from build123d import *

# Parameters (mm, degrees)
SKETCH1_R           = 14.2875
BOSS_EXTRUDE1_DEPTH = 11.1125
SKETCH2_R           = 15.875
BOSS_EXTRUDE2_DEPTH = 3.175
SKETCH3_R           = 6.35
CUT_EXTRUDE1_DEPTH  = 26.050327468


with BuildPart() as part:
    # Sketch1 → Boss-Extrude1 (new body)
    with BuildSketch(Plane(origin=(0, 0, 0), x_dir=(1, 0, 0), z_dir=(0, 1, 0))):
        with Locations(Location((0, 0, 0), (0, 0, 270))):
            Circle(SKETCH1_R)
    extrude(amount=BOSS_EXTRUDE1_DEPTH)

    # Sketch2 → Boss-Extrude2 (add)
    with BuildSketch(Plane(origin=(0, 11.1125, 0), x_dir=(1, 0, 0), z_dir=(0, 1, 0))):
        with Locations(Location((0, 0, 0), (0, 0, 270))):
            Circle(SKETCH2_R)
    extrude(amount=-BOSS_EXTRUDE2_DEPTH)

    # Sketch3 → Cut-Extrude1 (cut, through all)
    with BuildSketch(Plane(origin=(0, 11.1125, 0), x_dir=(1, 0, 0), z_dir=(0, 1, 0))):
        with Locations(Location((0, 0, 0), (0, 0, 270))):
            Circle(SKETCH3_R)
    extrude(amount=-CUT_EXTRUDE1_DEPTH, mode=Mode.SUBTRACT)


solid = part.part
Work out the finished part from the listing and answer in its coordinate system (mm). A direction names the side the tool comes from. Coordinates: 2 decimals unless noted, no trailing zeros. Write each loop counter-clockwise with the first axis right and the second up, starting at its lowest first coordinate (ties: lowest second). Pieces come first, ordered by that corner, then holes. Notation, with made-up numbers: M 22.25,40 L 67.25,40 A24 ccw 67.25,76 Z; hole C -40,24 d6. An arc over 180 degrees is marked long. Use one line per item in the form item = value. Start each with the question number.
1. Straight lines are drawn through the part: probe 1 along X at (y, z) = (7.25, 0); probe 2 along X at (y, z) = (8, 0) (3 decimals); probe 3 along Z at (x, y) = (3.5, 8.25). For each, find the intervals that lie inside material, in ascending order. Write a range as from..to.
2. The part is cut by section D-D (x = -7.5). Give the vertices of the cut face in (y, z).
3. The mould has two halves that part along Z. Classify faces 3 (the face through (-3.86, 5.63, -5.04)), 4 (the face through (-15.497, 9.547, -3.441)), 5 (the face through (-7, 11.112, 0)): released by +Z, released by -Z, zero draft, split by the parting line, or undercut.
4. Each of these flat-tipped pins is pushed along its axis until it touches: P1, Ø6, axis at x = 3.5, z = 3.5, coming from the -Y side; P2, Ø10, axis at x = 0, z = 0, coming from the -Y side; P3, Ø6, axis at x = 3.5, y = 6.5, coming from the -Z side; P4, Ø1, axis at y = 3, z = -11, coming from the +X side. Where does it stop, or does it pass through?
5. A tool of negligible diameter and unlimited length cuts with its end or side. For faces 1 (the face through (0.628, 3.913, -14.274)), 2 (the face through (-3, 0, 6)), from which of +Z, -Z, +X, -X, +Y, -Y can it reach the whole face along a straight path? Write none if from no direction.
6. The part is cut by section C-C (y = 10). Give the vertices of the cut face in (x, z) (3 decimals), plus the area to 3 significant figures.
Evaluation:
q1.probe_1 = -14.29..-6.35, 6.35..14.29
q1.probe_2 = -15.875..-6.35, 6.35..15.875
q1.probe_3 = -15.48..-5.3, 5.3..15.48
q2.outline = M 0,-12.16 L 7.94,-12.16 L 7.94,-13.99 L 11.11,-13.99 L 11.11,13.99 L 7.94,13.99 L 7.94,12.16 L 0,12.16 Z
q3.face_3 = undercut
q3.face_4 = split by the parting line
q3.face_5 = zero draft
q4.P1 = 0
q4.P2 = through
q4.P3 = -15.85
q4.P4 = 9.69
q5.face_1 = -Y
q5.face_2 = +Z, -Z, +X, -X, -Y
q6.outline = C 0,0 d31.75; hole C 0,0 d12.7
q6.area = 665 mm^2
